Can you work these out from the model? Positions are in its coordinate system, mm. A direction names the side the tool comes from. Give positions to 0.01 mm unless a question says otherwise; leave off trailing zeros. Order: outer loops, then holes, each group sorted by start corner. A loop starts at its lowest first (then second) coordinate and runs counter-clockwise, first axis right, second up. Notation, with made-up numbers: M -9.75,60.25 L 14.25,60.25 A25 ccw 14.25,83.25 Z; hole C -39.75,79.25 d10. An arc over 180 degrees is marked long. Answer as a JSON object with one key per item and string values.
```python
from build123d import *

# Parameters (mm, degrees)
SKETCH1_W              = 63
SKETCH1_H              = 63
BASE_PLATE_DEPTH       = 7
SKETCH4_W              = 34
SKETCH4_H              = 42.3
MAIN_SUPPORT_DEPTH     = 20
SKETCH5_W              = 12
SKETCH5_H              = 42.335
SCREW_SUPPORT_DEPTH    = 62.3
SKETCH6_R              = 12
SKETCH6_R_2            = 1.555
SCREW_DEPTH            = 50
SCREW_SUPPORT_FILLET_R = 5
BASE_SCREW_REACH       = 80.546
SKETCH7_R              = 1


with BuildPart() as part:
    # Sketch1 → Base Plate (new body)
    with BuildSketch(Plane(origin=(0, 0, 0), x_dir=(1, 0, 0), z_dir=(0, 1, 0))):
        with Locations((4.5, 0)):
            Rectangle(SKETCH1_W, SKETCH1_H)
    extrude(amount=BASE_PLATE_DEPTH)

    # Sketch4 → Main Support (add)
    with BuildSketch(Plane(origin=(0, 7, 0), x_dir=(1, 0, 0), z_dir=(0, 1, 0))):
        Rectangle(SKETCH4_W, SKETCH4_H)
    extrude(amount=MAIN_SUPPORT_DEPTH)

    # Sketch5 → Screw Support (add)
    with BuildSketch(Plane(origin=(0, 7, 0), x_dir=(1, 0, 0), z_dir=(0, 1, 0))):
        with Locations((23, -0.0175)):
            Rectangle(SKETCH5_W, SKETCH5_H)
    extrude(amount=SCREW_SUPPORT_DEPTH)

    # Sketch6 → Screw (cut)
    with BuildSketch(Plane(origin=(29, 0, 0), x_dir=(0, 0, -1), z_dir=(1, 0, 0))):
        with Locations((0, 48.15)):
            Circle(SKETCH6_R)
        with Locations((-15.5, 32.65)):
            Circle(SKETCH6_R_2)
        with Locations((15.5, 32.65)):
            Circle(SKETCH6_R_2)
        with Locations((15.5, 63.65)):
            Circle(SKETCH6_R_2)
        with Locations((-15.5, 63.65)):
            Circle(SKETCH6_R_2)
    extrude(amount=-SCREW_DEPTH, mode=Mode.SUBTRACT)

    # Screw Support Fillet
    screw_support_fillet_edges = [part.edges().sort_by_distance(p)[0] for p in [
        (23, 69.3, 21.185),
        (23, 69.3, -21.15),
    ]]
    fillet(screw_support_fillet_edges, radius=SCREW_SUPPORT_FILLET_R)

    # Sketch7 → Base Screw (cut, up to next)
    with BuildSketch(Plane(origin=(0, 7, 0), x_dir=(1, 0, 0), z_dir=(0, 1, 0)), mode=Mode.PRIVATE) as base_screw_sk1:
        with Locations(Location((-22, 26.5, 0), (0, 0, 270))):
            Circle(SKETCH7_R)
    base_screw_tool1 = extrude(base_screw_sk1.sketch, amount=-BASE_SCREW_REACH, mode=Mode.PRIVATE) & part.part
    # Sketch7 → Base Screw (cut, up to next)
    with BuildSketch(Plane(origin=(0, 7, 0), x_dir=(1, 0, 0), z_dir=(0, 1, 0)), mode=Mode.PRIVATE) as base_screw_sk2:
        with Locations(Location((31, 26.5, 0), (0, 0, 270))):
            Circle(SKETCH7_R)
    base_screw_tool2 = extrude(base_screw_sk2.sketch, amount=-BASE_SCREW_REACH, mode=Mode.PRIVATE) & part.part
    # Sketch7 → Base Screw (cut, up to next)
    with BuildSketch(Plane(origin=(0, 7, 0), x_dir=(1, 0, 0), z_dir=(0, 1, 0)), mode=Mode.PRIVATE) as base_screw_sk3:
        with Locations(Location((31, -26.5, 0), (0, 0, 270))):
            Circle(SKETCH7_R)
    base_screw_tool3 = extrude(base_screw_sk3.sketch, amount=-BASE_SCREW_REACH, mode=Mode.PRIVATE) & part.part
    # Sketch7 → Base Screw (cut, up to next)
    with BuildSketch(Plane(origin=(0, 7, 0), x_dir=(1, 0, 0), z_dir=(0, 1, 0)), mode=Mode.PRIVATE) as base_screw_sk4:
        with Locations(Location((-22, -26.5, 0), (0, 0, 270))):
            Circle(SKETCH7_R)
    base_screw_tool4 = extrude(base_screw_sk4.sketch, amount=-BASE_SCREW_REACH, mode=Mode.PRIVATE) & part.part
    add(base_screw_tool1.solids().sort_by_distance((-22, 7, -26.5))[0], mode=Mode.SUBTRACT)
    add(base_screw_tool2.solids().sort_by_distance((31, 7, -26.5))[0], mode=Mode.SUBTRACT)
    add(base_screw_tool3.solids().sort_by_distance((31, 7, 26.5))[0], mode=Mode.SUBTRACT)
    add(base_screw_tool4.solids().sort_by_distance((-22, 7, 26.5))[0], mode=Mode.SUBTRACT)


solid = part.part
```
1) For faces 1 (the face through (11, 23, -21.15)), 2 (the face through (29, 31, 0)), 3 (the face through (23, 35, 21.185)), 4 (the face through (4, 3, -31.5)), which set-ups out of +Z, -Z, +X, -X, +Y, -Y let a thin tool reach every point of the face, with its end or its side?
Results found:
{"face 1": "-Z, +X, -X, +Y", "face 2": "+Z, -Z, +X, +Y", "face 3": "+Z, +X, -X, +Y", "face 4": "-Z, +X, -X, +Y, -Y"}
2) I'm going to push flat-ended pins straight in: pin 1 Ø6 at (x, y) = (-0.5, 21.5) entering from +Z; pin 2 Ø8 at (y, z) = (48.5, -10) entering from -X; pin 3 Ø1.9 at (y, z) = (63.65, 15.5) entering from +X; pin 4 Ø17 at (x, z) = (-1, -5) entering from +Y. Where does each tip first touch, or does it pass through?
Results found:
{"pin 1": "stops at z = 21.15", "pin 2": "stops at x = 17", "pin 3": "passes through", "pin 4": "stops at y = 27"}
3) I want a section at A-A on z = -26.5. Write out the boundary of the cut face in (x, y), and give its area (3 significant figures).
Results found:
{"outline": "M -27,0 L -23,0 L -23,7 L -27,7 Z; M -21,0 L 30,0 L 30,7 L -21,7 Z; M 32,0 L 36,0 L 36,7 L 32,7 Z", "area": "413 mm²"}
4) I need wall thicknesses on L1, parallel to X at y = 3.5, z = -26.5; L2, parallel to Y at x = 22, z = -15.5 (3 decimals); L3, parallel to Z at x = 23, y = 32 (3 decimals). Which ranges of each line are inside material? Lowest first, please.
Results found:
{"L1": "x = -27 to -23, -21 to 30, 32 to 36", "L2": "y = 0 to 31.095, 34.205 to 62.095, 65.205 to 69.3", "L3": "z = -21.15 to -16.913, -14.087 to 14.087, 16.913 to 21.185"}
5) I want a section at B-B on y = 32.65. Write out the boundary of the cut face in (x, z) (3 decimals).
Results found:
{"outline": "M 17,-21.15 L 29,-21.15 L 29,-17.055 L 17,-17.055 Z; M 17,-13.945 L 29,-13.945 L 29,13.945 L 17,13.945 Z; M 17,17.055 L 29,17.055 L 29,21.185 L 17,21.185 Z"}
6) Thinking about a two-plate mould opening in Y: for faces 5 (the face through (0, 27, 0)), 6 (the face through (23.08, 60.05, 1.56)), 7 (the face through (-27, 3, 0)), which applies, pulls with the +Y half, pulls with the -Y half, needs draft (parallel to the pull), parting line crosses it, or undercut?
Results found:
{"face 5": "pulls with the +Y half", "face 6": "undercut", "face 7": "needs draft"}
7) I want a section at C-C on x = 25. Write out the boundary of the cut face in (y, z) (3 decimals).
Results found:
{"outline": "M 0,-31.5 L 7,-31.5 L 7,-21.15 L 64.3,-21.15 A5 ccw 69.3,-16.15 L 69.3,16.185 A5 ccw 64.3,21.185 L 7,21.185 L 7,31.5 L 0,31.5 Z; hole C 32.65,-15.5 d3.11; hole C 32.65,15.5 d3.11; hole C 48.15,0 d24; hole C 63.65,-15.5 d3.11; hole C 63.65,15.5 d3.11"}
8) I want a section at D-D on x = 11. Write out the boundary of the cut face in (y, z).
Results found:
{"outline": "M 0,-31.5 L 7,-31.5 L 7,-21.15 L 27,-21.15 L 27,21.15 L 7,21.15 L 7,31.5 L 0,31.5 Z"}
